Part model, mm, in its own coordinate system. A direction names the side the tool comes from. Give positions to 0.01 mm unless a question says otherwise; leave off trailing zeros. Order: outer loops, then holes, each group sorted by start corner. A loop starts at its lowest first (then second) coordinate and runs counter-clockwise, first axis right, second up. Notation, with made-up numbers: (-21, 6.25) - (29, 6.25) arc R20 ccw to (29, 41.25) - close; hole circle Ø7 at (-15.5, -31). An arc over 180 degrees is marked (long way). One line per item, written item: value.
```python
from build123d import *

# Parameters (mm, degrees)
SKETCH_1_W          = 50
SKETCH_1_H          = 55.5
EXTRUDE_1_DEPTH     = 60
SKETCH_3_W          = 50
SKETCH_3_H          = 53.5
CUT_EXTRUDE_1_DEPTH = 55
SKETCH_4_W          = 50
SKETCH_4_H          = 2
EXTRUDE_2_DEPTH     = 20
FILLET_5_R          = 1
SCALE_1_SCALE       = 1.7


with BuildPart() as part:
    # 草图1 → 凸台-拉伸1 (new body)
    with BuildSketch(Plane.XY):
        with Locations((6.818181818, -9.182037969)):
            Rectangle(SKETCH_1_W, SKETCH_1_H)
    extrude(amount=EXTRUDE_1_DEPTH)

    # 草图3 → 切除-拉伸1 (cut)
    with BuildSketch(Plane.XY.offset(60)):
        with Locations((6.818181818, -10.182037969)):
            Rectangle(SKETCH_3_W, SKETCH_3_H)
    extrude(amount=-CUT_EXTRUDE_1_DEPTH, mode=Mode.SUBTRACT)

    # 草图4 → 凸台-拉伸2 (add)
    with BuildSketch(Plane(origin=(0, 0, 0), x_dir=(-1, 0, 0), z_dir=(0, 0, -1))):
        with Locations((-6.818181818, -35.932037969)):
            Rectangle(SKETCH_4_W, SKETCH_4_H)
    extrude(amount=EXTRUDE_2_DEPTH)

    # 圆角5
    fillet_5_edges = [part.edges().sort_by_distance(p)[0] for p in [
        (6.818181818, 18.567962031, 60),
        (31.818181818, -8.182037969, 0),
        (6.818181818, -34.932037969, 0),
        (-18.181818182, -34.932037969, -10),
        (31.818181818, -34.932037969, -10),
        (6.818181818, 18.567962031, 0),
        (-18.181818182, -8.182037969, 0),
        (-18.181818182, 18.567962031, 30),
        (31.818181818, 18.567962031, 30),
    ]]
    fillet(fillet_5_edges, radius=FILLET_5_R)


with BuildPart() as part_1:
    # 缩放比例1: scaled about (0, 0, 0)
    add(part.part.scale(SCALE_1_SCALE))


solid = part_1.part
```
1) Slice it at A-A on x = 41. Write the cut outline in (y, z).
Answer:
outline: (-62.78, -34) - (-59.38, -34) - (-59.38, -1.7) arc R1.7 cw to (-57.68, 0) - (29.87, 0) arc R1.7 ccw to (31.57, 1.7) - (31.57, 100.3) arc R1.7 ccw to (29.87, 102) - (28.17, 102) - (28.17, 8.5) - (-62.78, 8.5) - close
2) Which spindle directions (+Z, -Z, +X, -X, +Y, -Y) get a long thin tool onto all of the face, cutting with end or side? Do faces 1 (the face through (11, -13, 0)), 2 (the face through (12, -61, -34)), 3 (the face through (11, -17, 8.5)). Say none if no direction does.
Answer:
face 1: -Z, +X, -X, +Y
face 2: -Z, +X, -X, +Y, -Y
face 3: +Z, +X, -X, -Y
3) Slice it at C-C on z = 39. Write the cut outline in (x, y).
Answer:
outline: (-30.91, 28.17) - (54.09, 28.17) - (54.09, 29.87) arc R1.7 ccw to (52.39, 31.57) - (-29.21, 31.57) arc R1.7 ccw to (-30.91, 29.87) - close
4) Drop flat-ended pins along their axis: P1, Ø1, axis at x = 10, z = 40, coming from the -Y side; P2, Ø6, axis at x = -9, y = -17, coming from the -Z side; P3, Ø2, axis at x = 37, y = -35, coming from the +Z side. Give the stop position or say it passes through.
Answer:
P1: stops at y = 28.17
P2: stops at z = 0
P3: stops at z = 8.5
5) Wall check: line 1 along Z through (x, y) = (40, -50); line 2 along Y through (x, z) = (0.5, -6.5); line 3 along Y through (x, z) = (-10, 57). Give the ranges that are in metal, low to high. Write a range as [from, to].
Answer:
line 1: z = [0, 8.5]
line 2: y = [-62.78, -59.38]
line 3: y = [28.17, 31.57]
6) Slice it at B-B on y = 8. Write the cut outline in (x, z).
Answer:
outline: (-30.91, 1.7) arc R1.7 ccw to (-29.21, 0) - (52.39, 0) arc R1.7 ccw to (54.09, 1.7) - (54.09, 8.5) - (-30.91, 8.5) - close
